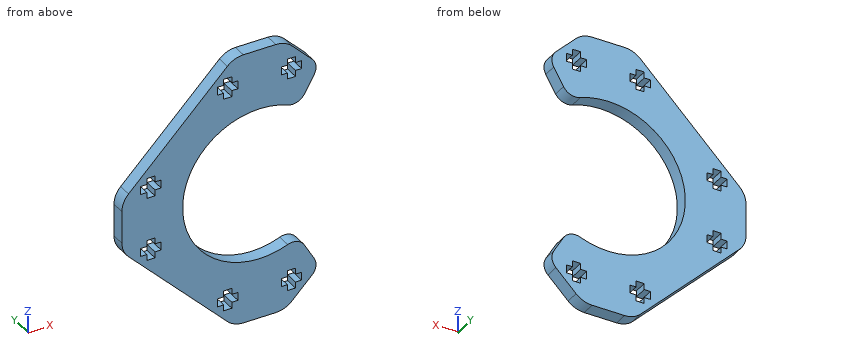
```python
from build123d import *

# Parameters (mm, degrees)
BOSS_EXTRUDE1_DEPTH = 3
CUT_EXTRUDE1_DEPTH  = 4
FILLET1_R           = 3


with BuildPart() as part:
    # Sketch1 → Boss-Extrude1 (new body)
    with BuildSketch(Plane(origin=(0, 0, 0), x_dir=(1, 0, 0), z_dir=(0, 1, 0))):
        with BuildLine():
            Line((17.56993863, 22.86267454), (11.491487674, 28.941125497))
            ThreePointArc((11.491487674, 28.941125497), (9.869370929, 30.024989254), (7.955953768, 30.405591591))
            Line((7.955953768, 30.405591591), (0.784380892, 30.405591591))
            ThreePointArc((0.784380892, 30.405591591), (-1.129036269, 30.024989254), (-2.751153014, 28.941125497))
            Line((-2.751153014, 28.941125497), (-24.570958167, 7.121320344))
            ThreePointArc((-24.570958167, 7.121320344), (-25.654821924, 5.499203599), (-26.035424261, 3.585786438))
            Line((-26.035424261, 3.585786438), (-26.035424261, -3.585786438))
            ThreePointArc((-26.035424261, -3.585786438), (-25.654821924, -5.499203599), (-24.570958167, -7.121320344))
            Line((-24.570958167, -7.121320344), (-2.751153014, -28.941125497))
            ThreePointArc((-2.751153014, -28.941125497), (-1.129036269, -30.024989254), (0.784380892, -30.405591591))
            Line((0.784380892, -30.405591591), (7.955953768, -30.405591591))
            ThreePointArc((7.955953768, -30.405591591), (9.869370929, -30.024989254), (11.491487674, -28.941125497))
            Line((11.491487674, -28.941125497), (17.56993863, -22.86267454))
            Line((17.56993863, -22.86267454), (12.87016733, -14.722431864))
            ThreePointArc((12.87016733, -14.722431864), (-12.62983267, 0), (12.87016733, 14.722431864))
            Line((12.87016733, 14.722431864), (17.56993863, 22.86267454))
        make_face()
    extrude(amount=BOSS_EXTRUDE1_DEPTH)

    # Sketch2 → Cut-Extrude1 (cut, through all)
    with BuildSketch(Plane(origin=(0, 3, 0), x_dir=(1, 0, 0), z_dir=(0, 1, 0))):
        Polygon((-21.87983267, 7.929437252), (-21.87983267, 6.129437252), (-20.52983267, 6.129437252), (-20.52983267, 4.779437252), (-18.72983267, 4.779437252), (-18.72983267, 6.129437252), (-17.37983267, 6.129437252), (-17.37983267, 7.929437252), (-18.72983267, 7.929437252), (-18.72983267, 9.279437252), (-20.52983267, 9.279437252), (-20.52983267, 7.929437252), align=None)
        Polygon((-18.72983267, -4.779437252), (-20.52983267, -4.779437252), (-20.52983267, -6.129437252), (-21.87983267, -6.129437252), (-21.87983267, -7.929437252), (-20.52983267, -7.929437252), (-20.52983267, -9.279437252), (-18.72983267, -9.279437252), (-18.72983267, -7.929437252), (-17.37983267, -7.929437252), (-17.37983267, -6.129437252), (-18.72983267, -6.129437252), align=None)
        Polygon((12.299604582, 23.1), (13.649604582, 23.1), (13.649604582, 24.9), (12.299604582, 24.9), (12.299604582, 26.25), (10.499604582, 26.25), (10.499604582, 24.9), (9.149604582, 24.9), (9.149604582, 23.1), (10.499604582, 23.1), (10.499604582, 21.75), (12.299604582, 21.75), align=None)
        Polygon((30.62016733, -7.929437252), (30.62016733, -6.129437252), (29.27016733, -6.129437252), (29.27016733, -4.779437252), (27.47016733, -4.779437252), (27.47016733, -6.129437252), (26.12016733, -6.129437252), (26.12016733, -7.929437252), (27.47016733, -7.929437252), (27.47016733, -9.279437252), (29.27016733, -9.279437252), (29.27016733, -7.929437252), align=None)
        Polygon((-0.409269922, 24.9), (-1.759269922, 24.9), (-1.759269922, 26.25), (-3.559269922, 26.25), (-3.559269922, 24.9), (-4.909269922, 24.9), (-4.909269922, 23.1), (-3.559269922, 23.1), (-3.559269922, 21.75), (-1.759269922, 21.75), (-1.759269922, 23.1), (-0.409269922, 23.1), align=None)
        Polygon((30.62016733, 7.929437252), (29.27016733, 7.929437252), (29.27016733, 9.279437252), (27.47016733, 9.279437252), (27.47016733, 7.929437252), (26.12016733, 7.929437252), (26.12016733, 6.129437252), (27.47016733, 6.129437252), (27.47016733, 4.779437252), (29.27016733, 4.779437252), (29.27016733, 6.129437252), (30.62016733, 6.129437252), align=None)
        Polygon((-1.759269922, -26.25), (-1.759269922, -24.9), (-0.409269922, -24.9), (-0.409269922, -23.1), (-1.759269922, -23.1), (-1.759269922, -21.75), (-3.559269922, -21.75), (-3.559269922, -23.1), (-4.909269922, -23.1), (-4.909269922, -24.9), (-3.559269922, -24.9), (-3.559269922, -26.25), align=None)
        Polygon((12.299604582, -26.25), (12.299604582, -24.9), (13.649604582, -24.9), (13.649604582, -23.1), (12.299604582, -23.1), (12.299604582, -21.75), (10.499604582, -21.75), (10.499604582, -23.1), (9.149604582, -23.1), (9.149604582, -24.9), (10.499604582, -24.9), (10.499604582, -26.25), align=None)
    extrude(amount=-CUT_EXTRUDE1_DEPTH, mode=Mode.SUBTRACT)

    # Fillet1
    fillet1_edges = [part.edges().sort_by_distance(p)[0] for p in [
        (12.87016733, 1.5, 14.722431864),
        (17.56993863, 1.5, 22.86267454),
        (17.56993863, 1.5, -22.86267454),
        (12.87016733, 1.5, -14.722431864),
    ]]
    fillet(fillet1_edges, radius=FILLET1_R)


solid = part.part
```
The listing builds one solid part. Answer for the finished solid, in the listing's coordinates (mm). Round coordinates to 2 decimals unless told otherwise and drop trailing zeros. Loops run counter-clockwise (first coordinate to the right, second up) from the corner with the lowest first, then second, coordinate; pieces in that order, holes last. Notation, with made-up numbers: (74, -39) - (80, -39) arc R25 ccw to (80, -27) - close; hole circle Ø4 at (21.5, 23.25). An arc over 180 degrees is marked (long way). Return JSON: item names as keys, results as strings. Group by question number.
1. The part is cut by section A-A on x = 6.5. Determine the outline of the cut face in (y, z), then the cut area to 3 significant figures.
2. Consider probe 1 along Z at (x, y) = (5, 1.7); probe 2 along Z at (x, y) = (-4.5, 0.6); probe 3 along Z at (x, y) = (-6, 0.4). Determine where each line is inside the solid, lowest interval first.
3. The part is cut by section C-C on z = 0. Determine the outline of the cut face in (x, y), then the cut area to 3 significant figures.
4. Each of these flat-tipped pins is pushed along its axis until it touches: P1, Ø1.1, axis at y = 1.5, z = 5.5, coming from the +X side; P2, Ø0.9, axis at x = -3, y = 1.5, coming from the -Z side; P3, Ø0.9, axis at y = 1.5, z = -24, coming from the +X side. Where does it stop, or does it pass through?
5. The part is cut by section D-D on y = 2.3. State how many separate pieces and enclosed holes the cut face has, then the cut area to 3 significant figures.
6. The part is cut by section B-B on x = -19.5. Determine the outline of the cut face in (y, z).
Resolved:
{
 "1": {"outline": "(0, -30.41) - (3, -30.41) - (3, -16.87) - (0, -16.87) - close; (0, 16.87) - (3, 16.87) - (3, 30.41) - (0, 30.41) - close", "area": "81.2 mm²"},
 "2": {"probe 1": "z = -30.41 to -16.99, 16.99 to 30.41", "probe 2": "z = -27.19 to -24.9, -23.1 to -14.5, 14.5 to 23.1, 24.9 to 27.19", "probe 3": "z = -25.69 to -13.47, 13.47 to 25.69"},
 "3": {"outline": "(-26.04, 0) - (-12.63, 0) - (-12.63, 3) - (-26.04, 3) - close", "area": "40.2 mm²"},
 "4": {"P1": "stops at x = -11.52", "P2": "stops at z = -29.13", "P3": "stops at x = 16.58"},
 "5": {"separate pieces": "1", "enclosed holes": "6", "area": "989 mm²"},
 "6": {"outline": "(0, -12.19) - (3, -12.19) - (3, -9.28) - (0, -9.28) - close; (0, -4.78) - (3, -4.78) - (3, 4.78) - (0, 4.78) - close; (0, 9.28) - (3, 9.28) - (3, 12.19) - (0, 12.19) - close"}
}
